```python
from build123d import *

# Parameters (mm, degrees)
SKETCH1_W                      = 20
SKETCH1_H                      = 50
BOSS_EXTRUDE1_DEPTH            = 12
CUT_EXTRUDE1_REACH             = 54.383
SKETCH4_W                      = 50
SKETCH4_H                      = 9.5
BOSS_EXTRUDE2_DEPTH            = 14.5
SKETCH5_W                      = 50
SKETCH5_H                      = 9.5
BOSS_EXTRUDE3_DEPTH            = 14.5
SKETCH10_R                     = 5
CUT_EXTRUDE4_DEPTH             = 7
CUT_EXTRUDE4_DIRECTION_2_REACH = 38.27
CUT_EXTRUDE5_REACH             = 38.27
SKETCH11_R                     = 2.25


with BuildPart() as part:
    # Sketch1 → Boss-Extrude1 (new body)
    with BuildSketch(Plane(origin=(0, 0, 0), x_dir=(1, 0, 0), z_dir=(0, 1, 0))):
        Rectangle(SKETCH1_W, SKETCH1_H)
    extrude(amount=BOSS_EXTRUDE1_DEPTH)

    # Sketch2 → Cut-Extrude1 (cut, up to next)
    with BuildSketch(Plane.XY.offset(25), mode=Mode.PRIVATE) as cut_extrude1_sk1:
        Polygon((0, 9.5), (7.25, 9.5), (6.25, 12), (0, 12), (-6.25, 12), (-7.25, 9.5), align=None)
    cut_extrude1_tool1 = extrude(cut_extrude1_sk1.sketch, amount=-CUT_EXTRUDE1_REACH, mode=Mode.PRIVATE) & part.part
    add(cut_extrude1_tool1.solids().sort_by_distance((0, 10.719136, 25))[0], mode=Mode.SUBTRACT)

    # Sketch4 → Boss-Extrude2 (add)
    with BuildSketch(Plane.ZY.offset(10)):
        with Locations((0, 4.75)):
            Rectangle(SKETCH4_W, SKETCH4_H)
    extrude(amount=BOSS_EXTRUDE2_DEPTH)

    # Sketch5 → Boss-Extrude3 (add)
    with BuildSketch(Plane(origin=(10, 0, 0), x_dir=(0, 0, -1), z_dir=(1, 0, 0))):
        with Locations((0, 4.75)):
            Rectangle(SKETCH5_W, SKETCH5_H)
    extrude(amount=BOSS_EXTRUDE3_DEPTH)

    # Sketch10 → Cut-Extrude4 (cut)
    with BuildSketch(Plane(origin=(0, 9.5, 0), x_dir=(1, 0, 0), z_dir=(0, 1, 0))):
        with Locations(Location((-12.5, 12.5, 0), (0, 0, 60))):
            Circle(SKETCH10_R)
        with Locations(Location((12.5, 12.5, 0), (0, 0, 120))):
            Circle(SKETCH10_R)
        with Locations(Location((-12.5, -12.5, 0), (0, 0, 60))):
            Circle(SKETCH10_R)
        with Locations(Location((12.5, -12.5, 0), (0, 0, 120))):
            Circle(SKETCH10_R)
    extrude(amount=-CUT_EXTRUDE4_DEPTH, mode=Mode.SUBTRACT)

    # Sketch10 → Cut-Extrude4 direction 2 (cut, up to next)
    with BuildSketch(Plane(origin=(0, 9.5, 0), x_dir=(1, 0, 0), z_dir=(0, 1, 0)), mode=Mode.PRIVATE) as cut_extrude4_direction_2_sk1:
        with Locations(Location((-12.5, 12.5, 0), (0, 0, 60))):
            Circle(SKETCH10_R)
    cut_extrude4_direction_2_tool1 = extrude(cut_extrude4_direction_2_sk1.sketch, amount=CUT_EXTRUDE4_DIRECTION_2_REACH, mode=Mode.PRIVATE) & part.part
    # Sketch10 → Cut-Extrude4 direction 2 (cut, up to next)
    with BuildSketch(Plane(origin=(0, 9.5, 0), x_dir=(1, 0, 0), z_dir=(0, 1, 0)), mode=Mode.PRIVATE) as cut_extrude4_direction_2_sk2:
        with Locations(Location((12.5, 12.5, 0), (0, 0, 120))):
            Circle(SKETCH10_R)
    cut_extrude4_direction_2_tool2 = extrude(cut_extrude4_direction_2_sk2.sketch, amount=CUT_EXTRUDE4_DIRECTION_2_REACH, mode=Mode.PRIVATE) & part.part
    # Sketch10 → Cut-Extrude4 direction 2 (cut, up to next)
    with BuildSketch(Plane(origin=(0, 9.5, 0), x_dir=(1, 0, 0), z_dir=(0, 1, 0)), mode=Mode.PRIVATE) as cut_extrude4_direction_2_sk3:
        with Locations(Location((-12.5, -12.5, 0), (0, 0, 60))):
            Circle(SKETCH10_R)
    cut_extrude4_direction_2_tool3 = extrude(cut_extrude4_direction_2_sk3.sketch, amount=CUT_EXTRUDE4_DIRECTION_2_REACH, mode=Mode.PRIVATE) & part.part
    # Sketch10 → Cut-Extrude4 direction 2 (cut, up to next)
    with BuildSketch(Plane(origin=(0, 9.5, 0), x_dir=(1, 0, 0), z_dir=(0, 1, 0)), mode=Mode.PRIVATE) as cut_extrude4_direction_2_sk4:
        with Locations(Location((12.5, -12.5, 0), (0, 0, 120))):
            Circle(SKETCH10_R)
    cut_extrude4_direction_2_tool4 = extrude(cut_extrude4_direction_2_sk4.sketch, amount=CUT_EXTRUDE4_DIRECTION_2_REACH, mode=Mode.PRIVATE) & part.part
    add(cut_extrude4_direction_2_tool1.solids().sort_by_distance((-12.5, 9.5, -12.5))[0], mode=Mode.SUBTRACT)
    add(cut_extrude4_direction_2_tool2.solids().sort_by_distance((12.5, 9.5, -12.5))[0], mode=Mode.SUBTRACT)
    add(cut_extrude4_direction_2_tool3.solids().sort_by_distance((-12.5, 9.5, 12.5))[0], mode=Mode.SUBTRACT)
    add(cut_extrude4_direction_2_tool4.solids().sort_by_distance((12.5, 9.5, 12.5))[0], mode=Mode.SUBTRACT)

    # Sketch11 → Cut-Extrude5 (cut, up to next)
    with BuildSketch(Plane(origin=(0, 2.5, 0), x_dir=(1, 0, 0), z_dir=(0, 1, 0)), mode=Mode.PRIVATE) as cut_extrude5_sk1:
        with Locations(Location((-12.5, 12.5, 0), (0, 0, 270))):
            Circle(SKETCH11_R)
    cut_extrude5_tool1 = extrude(cut_extrude5_sk1.sketch, amount=-CUT_EXTRUDE5_REACH, mode=Mode.PRIVATE) & part.part
    # Sketch11 → Cut-Extrude5 (cut, up to next)
    with BuildSketch(Plane(origin=(0, 2.5, 0), x_dir=(1, 0, 0), z_dir=(0, 1, 0)), mode=Mode.PRIVATE) as cut_extrude5_sk2:
        with Locations(Location((12.5, 12.5, 0), (0, 0, 270))):
            Circle(SKETCH11_R)
    cut_extrude5_tool2 = extrude(cut_extrude5_sk2.sketch, amount=-CUT_EXTRUDE5_REACH, mode=Mode.PRIVATE) & part.part
    # Sketch11 → Cut-Extrude5 (cut, up to next)
    with BuildSketch(Plane(origin=(0, 2.5, 0), x_dir=(1, 0, 0), z_dir=(0, 1, 0)), mode=Mode.PRIVATE) as cut_extrude5_sk3:
        with Locations(Location((-12.5, -12.5, 0), (0, 0, 270))):
            Circle(SKETCH11_R)
    cut_extrude5_tool3 = extrude(cut_extrude5_sk3.sketch, amount=-CUT_EXTRUDE5_REACH, mode=Mode.PRIVATE) & part.part
    # Sketch11 → Cut-Extrude5 (cut, up to next)
    with BuildSketch(Plane(origin=(0, 2.5, 0), x_dir=(1, 0, 0), z_dir=(0, 1, 0)), mode=Mode.PRIVATE) as cut_extrude5_sk4:
        with Locations(Location((12.5, -12.5, 0), (0, 0, 270))):
            Circle(SKETCH11_R)
    cut_extrude5_tool4 = extrude(cut_extrude5_sk4.sketch, amount=-CUT_EXTRUDE5_REACH, mode=Mode.PRIVATE) & part.part
    add(cut_extrude5_tool1.solids().sort_by_distance((-12.5, 2.5, -12.5))[0], mode=Mode.SUBTRACT)
    add(cut_extrude5_tool2.solids().sort_by_distance((12.5, 2.5, -12.5))[0], mode=Mode.SUBTRACT)
    add(cut_extrude5_tool3.solids().sort_by_distance((-12.5, 2.5, 12.5))[0], mode=Mode.SUBTRACT)
    add(cut_extrude5_tool4.solids().sort_by_distance((12.5, 2.5, 12.5))[0], mode=Mode.SUBTRACT)


solid = part.part
```
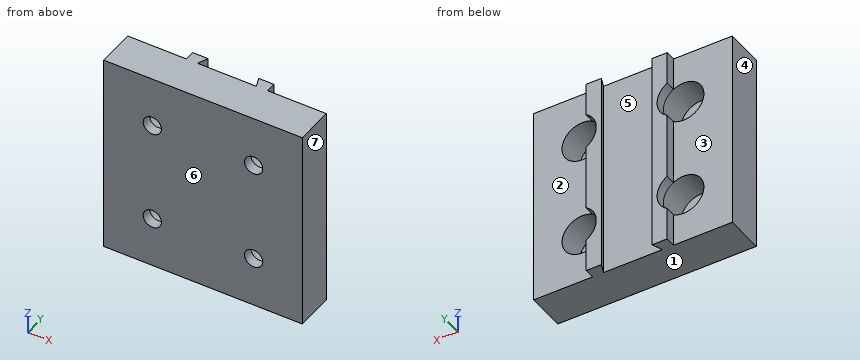
The listing builds one solid part. Answer for the finished solid, in the listing's coordinates (mm). Face numbers are marked on the shaded views. A direction names the side the tool comes from. Give positions to 0.01 mm unless a question says otherwise; leave off trailing zeros. Order: outer loops, then holes, each group sorted by start corner. A loop starts at its lowest first (then second) coordinate and runs counter-clockwise, first axis right, second up. Notation, with made-up numbers: M 51.5,-37.5 L 90.5,-37.5 A24 ccw 90.5,-23.5 Z; hole C 13,85.25 d2. An arc over 180 degrees is marked long. Put each result on its own line as item: value. Start each with the question number.
Item 1: The part is cut by section B-B, the plane z = 12.5. Determine the outline of the cut face in (x, y).
Item 2: Flat-ended cylindrical pins translate along their axes: P1, Ø5, axis at x = 13.5, z = -15, coming from the +Y side; P2, Ø3.5, axis at x = 12.5, z = -12.5, coming from the -Y side; P3, Ø3, axis at x = 13.5, z = 12.5, coming from the +Y side; P4, Ø2, axis at y = 11, z = 19, coming from the +X side. Find the tip coordinate at first contact, or state that the pin passes through.
Item 3: Which of the six approach directions +Z, -Z, +X, -X, +Y, -Y give full straight-line access (tool end or side, diameter ignored) to the marked faces 1, 2 and 3?
Item 4: The part is cut by section C-C, the plane x = 12.5. Determine the outline of the cut face in (y, z).
Item 5: The part is cut by section A-A, the plane y = 10.5. Determine the outline of the cut face in (x, z), and give its area (3 significant figures).
Item 6: The part is cut by section D-D, the plane y = 5. Determine the outline of the cut face in (x, z).
Item 7: Find the intervals of material crossed by line 1 along Z through (x, y) = (-12.5, 7); line 2 along X through (y, z) = (6, 10); line 3 along X through (y, z) = (1.8, 12.5), in increasing order.
Item 8: For a pull along X with two mould halves and no side action, classify the marked faces 4, 5, 6 and 7 as +X half, -X half, draft (parallel to the pull), parting line (faces both ways), or undercut.
Answer key:
1. outline: M -24.5,0 L -14.75,0 L -14.75,2.5 L -17.5,2.5 L -17.5,9.5 L -24.5,9.5 Z; M -10.25,0 L 10.25,0 L 10.25,2.5 L 7.5,2.5 L 7.5,12 L 6.25,12 L 7.25,9.5 L -7.25,9.5 L -6.25,12 L -7.5,12 L -7.5,2.5 L -10.25,2.5 Z; M 14.75,0 L 24.5,0 L 24.5,9.5 L 17.5,9.5 L 17.5,2.5 L 14.75,2.5 Z
2. P1: stops at y = 9.5
2. P2: passes through
2. P3: stops at y = 2.5
2. P4: stops at x = 10
3. face 1: -Z, +X, -X, +Y, -Y
3. face 2: +Z, -Z, +X, +Y
3. face 3: +Z, -Z, -X, +Y
4. outline: M 0,-25 L 9.5,-25 L 9.5,-17.5 L 2.5,-17.5 L 2.5,-14.75 L 0,-14.75 Z; M 0,-10.25 L 2.5,-10.25 L 2.5,-7.5 L 9.5,-7.5 L 9.5,7.5 L 2.5,7.5 L 2.5,10.25 L 0,10.25 Z; M 0,14.75 L 2.5,14.75 L 2.5,17.5 L 9.5,17.5 L 9.5,25 L 0,25 Z
5. outline: M -10,-25 L -6.85,-25 L -6.85,25 L -10,25 L -10,16.83 A5 cw -10,8.17 L -10,-8.17 A5 cw -10,-16.83 Z; M 6.85,-25 L 10,-25 L 10,-16.83 A5 cw 10,-8.17 L 10,8.17 A5 cw 10,16.83 L 10,25 L 6.85,25 Z
5. area: 254 mm²
6. outline: M -24.5,-25 L 24.5,-25 L 24.5,25 L -24.5,25 Z; hole C -12.5,-12.5 d10; hole C -12.5,12.5 d10; hole C 12.5,-12.5 d10; hole C 12.5,12.5 d10
7. line 1: z = -25 to -17.5, -7.5 to 7.5, 17.5 to 25
7. line 2: x = -24.5 to -16.83, -8.17 to 8.17, 16.83 to 24.5
7. line 3: x = -24.5 to -14.75, -10.25 to 10.25, 14.75 to 24.5
8. face 4: -X half
8. face 5: undercut
8. face 6: draft
8. face 7: +X half
